Autodesk Inventor part; units mm, degrees
ref_plane "YZ Plane" through (0, 0, 0) normal (1, 0, 0) x (0, 1, 0)
ref_plane "XZ Plane" through (0, 0, 0) normal (0, 1, 0) x (-1, 0, 0)
ref_plane "XY Plane" through (0, 0, 0) normal (0, 0, 1) x (1, 0, 0)
sketch "Sketch1" plane through (0, 0, 0) normal (0, 0, 1) x (1, 0, 0)
  line L0 (0, 0) -> (25.4, 0)
  line L1 (25.4, 0) -> (25.4, 50.8)
  line L2 (25.4, 50.8) -> (0, 50.8)
  line L3 (0, 50.8) -> (0, 0)
  dimension "d0" = 25.4
  dimension "d1" = 50.8
extrude "Extrusion1" add sketch "Sketch1" along normal blind 304.8
shell "Shell1" thickness 3.175 removed faces 2 at (8.4667, 33.8667, 0) at (8.4667, 33.8667, 304.8)
sketch "Sketch2" plane through (25.4, 0, 0) normal (1, 0, 0) x (0, 0, -1)
  line L0 (-304.8, 50.8) -> (-304.8, 0)
  line L1 (0, 50.8) -> (-304.8, 50.8)
  circle A0 centre (-292.1, 38.1) radius 2.3813
  dimension "d5" = 4.7625
  dimension "d6" = 12.7
  dimension "d7" = 12.7
extrude "Extrusion2" cut sketch "Sketch2" against normal through all
pattern_linear "Rectangular Pattern1" count 12 spacing 25.4 along (0, 0, -1) count 2 spacing 25.4 along (0, -1, 0) of "Extrusion2"
sketch "Sketch3" plane through (0, 50.8, 0) normal (0, 1, 0) x (1, 0, 0)
  line L0 (0, -304.8) -> (25.4, -304.8)
  line L1 (25.4, 0) -> (25.4, -304.8)
  line L2 (0, -304.8) -> (25.4, -304.8)
  line L3 (25.4, -254) -> (0, -304.8)
  dimension "d16" = 50.8
extrude "Extrusion3" cut sketch "Sketch3" against normal through all
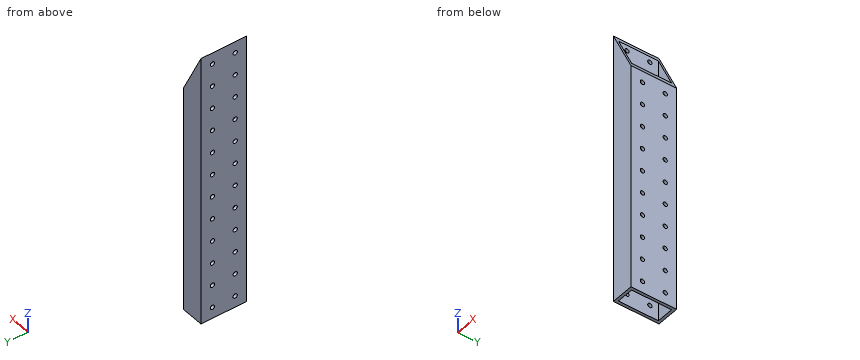
Model file for the job. Use its own axes, mm. Round coordinates to 2 decimals unless told otherwise and drop trailing zeros. Order: outer loops, then holes, each group sorted by start corner. A loop starts at its lowest first (then second) coordinate and runs counter-clockwise, first axis right, second up. Notation, with made-up numbers: M -37,-2 L -14,-2 A30 cw -14,30 Z; hole C 43,68.5 d7. An arc over 180 degrees is marked long. Use CSV: the item, a comma, the result in double quotes.
Item 1: Probe probe 1 along Y at (x, z) = (1.6, 12.7); probe 2 along X at (y, z) = (24.5, 42) (3 decimals); probe 3 along Y at (x, z) = (6.5, 83.5) (3 decimals). List the from-to ranges inside material, lowest first.
Worked answers:
probe 1,"0 to 10.32, 15.08 to 35.72, 40.48 to 50.8"
probe 2,"0 to 3.175, 22.225 to 25.4"
probe 3,"0 to 3.175, 47.625 to 50.8"
Item 2: Saw through at C-C (z = 100.5). List the corners of the cut face in (x, y) (3 decimals), plus the area to 3 significant figures.
Worked answers:
outline,"M 0,0 L 25.4,0 L 25.4,50.8 L 0,50.8 Z; hole M 3.175,3.175 L 22.225,3.175 L 22.225,47.625 L 3.175,47.625 Z"
area,"444 mm²"
Item 3: Saw through at A-A (x = 14.5). List the corners of the cut face in (y, z) (3 decimals), plus the area to 3 significant figures.
Worked answers:
outline,"M 0,0 L 3.175,0 L 3.175,275.8 L 0,275.8 Z; M 47.625,0 L 50.8,0 L 50.8,275.8 L 47.625,275.8 Z"
area,"1,750 mm²"
Item 4: Saw through at B-B (y = 23). List the corners of the cut face in (x, z) (3 decimals), plus the area to 3 significant figures.
Worked answers:
outline,"M 0,0 L 3.175,0 L 3.175,298.45 L 0,304.8 Z; M 22.225,0 L 25.4,0 L 25.4,254 L 22.225,260.35 Z"
area,"1,770 mm²"
